from build123d import *

# Parameters (mm, degrees)
SKETCH1_W               = 12.04
SKETCH1_H               = 7.58
SKETCH1_W_2             = 8.04
SKETCH1_H_2             = 3.58
BOSS_EXTRUDE1_DEPTH     = 8
SKETCH1_2_W             = 12.04
SKETCH1_2_H             = 7.58
SKETCH1_2_W_2           = 8.04
SKETCH1_2_H_2           = 3.58
BOSS_EXTRUDE2_DEPTH     = 2
EXTRUDE_THIN1_START     = -12.04
EXTRUDE_THIN1_DEPTH     = 12.04
SKETCH5_W               = 12.04
SKETCH5_H               = 7.58
SKETCH5_W_2             = 8.04
SKETCH5_H_2             = 3.58
BOSS_EXTRUDE4_DEPTH     = 10
SKETCH5_4_W             = 12.04
SKETCH5_4_H             = 7.58
BOSS_EXTRUDE5_DEPTH     = 2
CHAMFER1_SIZE           = 1.5
CUT_EXTRUDE1_DEPTH      = 31.858817668
CUT_EXTRUDE1_DEPTH_BACK = 31.858817668
CUT_EXTRUDE2_DEPTH      = 31.883619629
CUT_EXTRUDE2_DEPTH_BACK = 31.883619629
SKETCH8_W               = 4
SKETCH8_H               = 1.58
CUT_EXTRUDE3_DEPTH      = 7
SKETCH9_W               = 4
SKETCH9_H               = 1.58
CUT_EXTRUDE4_DEPTH      = 7
CHAMFER2_SIZE           = 0.5
BOSS_EXTRUDE6_DEPTH     = 0.3


with BuildPart() as part:
    # Sketch1 → Boss-Extrude1 (new body)
    with BuildSketch(Plane.XY):
        Rectangle(SKETCH1_W, SKETCH1_H)
        Rectangle(SKETCH1_W_2, SKETCH1_H_2, mode=Mode.SUBTRACT)
    extrude(amount=BOSS_EXTRUDE1_DEPTH)

    # Sketch1<2> → Boss-Extrude2 (add)
    # profile 1 of 2: a face of its own
    with BuildSketch(Plane.XY):
        Rectangle(SKETCH1_2_W, SKETCH1_2_H)
        Rectangle(SKETCH1_2_W_2, SKETCH1_2_H_2, mode=Mode.SUBTRACT)
    # profile 2 of 2: a face of its own
    with BuildSketch(Plane.XY):
        Rectangle(SKETCH1_2_W_2, SKETCH1_2_H_2)
    extrude(amount=-BOSS_EXTRUDE2_DEPTH)

    # Sketch3 → Extrude-Thin1 (add)
    with BuildSketch(Plane(origin=(6.02, 9.81, 0), x_dir=(0, -1, 0), z_dir=(1, 0, 0)).offset(EXTRUDE_THIN1_START)):
        with BuildLine():
            Line((13.6, 2), (9.52, 2))
            ThreePointArc((9.52, 2), (9.33452957, 10.5), (8.778471331, 18.983819807))
            Line((8.778471331, 18.983819807), (12.842945699, 19.339415237))
            Line((12.842945699, 19.339415237), (12.668634214, 21.331804633))
            Line((12.668634214, 21.331804633), (6.601440048, 20.800993925))
            ThreePointArc((6.601440048, 20.800993925), (7.336433126, 10.412761225), (7.509629919, 0))
            Line((7.509629919, 0), (13.6, 0))
            Line((13.6, 0), (13.6, 2))
        make_face()
    extrude(amount=EXTRUDE_THIN1_DEPTH)

    # Sketch5 → Boss-Extrude4 (add)
    with BuildSketch(Plane(origin=(0, -2.094837633, -19.257341416), x_dir=(-1, 0, 0), z_dir=(0, 0.08715574274765182, -0.9961946980917462))):
        with Locations((0, 2.848308513)):
            Rectangle(SKETCH5_W, SKETCH5_H)
        with Locations((0, 2.848308513)):
            Rectangle(SKETCH5_W_2, SKETCH5_H_2, mode=Mode.SUBTRACT)
    extrude(amount=BOSS_EXTRUDE4_DEPTH)

    # Sketch5<4> → Boss-Extrude5 (add)
    with BuildSketch(Plane(origin=(0, -2.094837633, -19.257341416), x_dir=(-1, 0, 0), z_dir=(0, 0.08715574274765182, -0.9961946980917462))):
        with Locations((0, 2.848308513)):
            Rectangle(SKETCH5_4_W, SKETCH5_4_H)
    extrude(amount=BOSS_EXTRUDE5_DEPTH)

    # Chamfer1
    chamfer1_edges = [part.edges().sort_by_distance(p)[0] for p in [
        (0, -3.79, -2),
        (0, 3.79, -2),
        (-6.02, -2.597166986, -24.320388728),
        (6.02, -2.597166986, -24.320388728),
        (0, -3.032945699, -19.339415237),
        (6.02, -3.79, 3),
        (-6.02, -3.79, 3),
        (-6.02, 3.79, 3),
        (6.02, 3.79, 3),
        (0, 4.518210112, -18.678774707),
        (6.02, 4.953988826, -23.659748198),
        (-6.02, 4.953988826, -23.659748198),
    ]]
    chamfer(chamfer1_edges, length=CHAMFER1_SIZE - 0.0001)  # a hair under: the kernel refuses the full size

    # Sketch6 → Cut-Extrude1 (cut, two sides: drawn at the far end of the back side and taken through both)
    with BuildSketch(Plane(origin=(0, 3.79, 0), x_dir=(1, 0, 0), z_dir=(0, 1, 0)).offset(-CUT_EXTRUDE1_DEPTH_BACK)):
        with BuildLine():
            Line((1.45, -3.566987298), (-0.35, -2.527756814))
            ThreePointArc((-0.35, -2.527756814), (-0.85, -2.527756814), (-1.1, -2.960769515))
            Line((-1.1, -2.960769515), (-1.1, -5.039230485))
            ThreePointArc((-1.1, -5.039230485), (-0.85, -5.472243186), (-0.35, -5.472243186))
            Line((-0.35, -5.472243186), (1.45, -4.433012702))
            ThreePointArc((1.45, -4.433012702), (1.7, -4), (1.45, -3.566987298))
        make_face()
    extrude(amount=CUT_EXTRUDE1_DEPTH + CUT_EXTRUDE1_DEPTH_BACK, mode=Mode.SUBTRACT)

    # Sketch7 → Cut-Extrude2 (cut, two sides: drawn at the far end of the back side and taken through both)
    with BuildSketch(Plane(origin=(0, 2.862121636, 0.250403197), x_dir=(1, 0, 0), z_dir=(0, 0.9961946980917462, 0.08715574274765181)).offset(-CUT_EXTRUDE2_DEPTH_BACK)):
        with BuildLine():
            Line((1.45, 25.43449699), (-0.35, 26.473727475))
            ThreePointArc((-0.35, 26.473727475), (-0.85, 26.473727475), (-1.1, 26.040714773))
            Line((-1.1, 26.040714773), (-1.1, 23.962253804))
            ThreePointArc((-1.1, 23.962253804), (-0.85, 23.529241102), (-0.35, 23.529241102))
            Line((-0.35, 23.529241102), (1.45, 24.568471587))
            ThreePointArc((1.45, 24.568471587), (1.7, 25.001484288), (1.45, 25.43449699))
        make_face()
    extrude(amount=CUT_EXTRUDE2_DEPTH + CUT_EXTRUDE2_DEPTH_BACK, mode=Mode.SUBTRACT)

    # Sketch8 → Cut-Extrude3 (cut)
    with BuildSketch(Plane(origin=(0, 2.527645904, -28.891124885), x_dir=(-1, 0, 0), z_dir=(0, 0.08715574274765193, -0.9961946980917461))):
        with Locations((-6.02, -0.916945525)):
            Rectangle(SKETCH8_W, SKETCH8_H)
    extrude(amount=-CUT_EXTRUDE3_DEPTH, mode=Mode.SUBTRACT)

    # Sketch9 → Cut-Extrude4 (cut)
    with BuildSketch(Plane.XY.offset(8)):
        with Locations((6.02, 0)):
            Rectangle(SKETCH9_W, SKETCH9_H)
    extrude(amount=-CUT_EXTRUDE4_DEPTH, mode=Mode.SUBTRACT)

    # Chamfer2
    chamfer2_edges = [part.edges().sort_by_distance(p)[0] for p in [
        (4.02, 0.522150723, -25.553213547),
        (4.02, 1.004099435, -21.997679067),
        (4.02, 2.096138346, -25.415507473),
        (4.02, 0.79, 4.5),
        (4.02, 0, 1),
        (4.02, -0.79, 4.5),
    ]]
    chamfer(chamfer2_edges, length=CHAMFER2_SIZE)

    # Sketch10 → Boss-Extrude6 (add)
    with BuildSketch(Plane(origin=(6.02, 0, 0), x_dir=(0, 0, -1), z_dir=(1, 0, 0))):
        with BuildLine():
            Line((21.338592032, 0.15320422), (21.233028007, 1.362426781))
            add(Edge.make_bspline(
                [(21.233028007, 1.362426781), (21.230623172, 1.392016851), (21.22550753, 1.454961769), (21.219940858, 1.554962176), (21.215964545, 1.666017285), (21.21390718, 1.743649504), (21.212829837, 1.784301781)],
                knots=[0, 0, 0, 0, 0.843314449, 1.793924683, 2.844783983, 4, 4, 4, 4], degree=3))
            Line((21.212829837, 1.784301781), (21.202540203, 1.783539585))
            add(Edge.make_bspline(
                [(21.202540203, 1.783539585), (21.200808847, 1.76790896), (21.197498896, 1.738026826), (21.192026096, 1.695375149), (21.187181442, 1.656725646), (21.182258815, 1.622035938), (21.177293915, 1.591439333), (21.172767869, 1.564856175), (21.168316369, 1.542328609), (21.164861999, 1.528700708), (21.163287154, 1.522487756)],
                knots=[0, 0, 0, 0, 1.428769924, 2.731477, 3.906784307, 4.967723303, 5.914548028, 6.722864751, 7.417754754, 8, 8, 8, 8], degree=3))
            Line((21.163287154, 1.522487756), (20.792098129, 0.105567024))
            Line((20.792098129, 0.105567024), (20.453683495, 0.075841415))
            Line((20.453683495, 0.075841415), (19.837067642, 1.393295683))
            add(Edge.make_bspline(
                [(19.837067642, 1.393295683), (19.835006874, 1.398111338), (19.83016149, 1.409434157), (19.822671636, 1.429138703), (19.813894021, 1.454208796), (19.803667873, 1.484424749), (19.792311733, 1.520061222), (19.779237689, 1.560762892), (19.765280196, 1.6069604), (19.755390982, 1.639486413), (19.750177398, 1.656634098)],
                knots=[0, 0, 0, 0, 0.453127431, 1.065416844, 1.823166036, 2.751085321, 3.825012516, 5.058876589, 6.449442438, 8, 8, 8, 8], degree=3))
            Line((19.750177398, 1.656634098), (19.738744471, 1.655490805))
            add(Edge.make_bspline(
                [(19.738744471, 1.655490805), (19.751035456, 1.572245864), (19.77562146, 1.405728657), (19.791432277, 1.238150394), (19.799338983, 1.154347512)],
                knots=[0, 0, 0, 0, 0.999835902, 2, 2, 2, 2], degree=3))
            Line((19.799338983, 1.154347512), (19.898043251, 0.027442024))
            Line((19.898043251, 0.027442024), (19.514659105, -0.006094561))
            Line((19.514659105, -0.006094561), (19.34049752, 1.986283488))
            Line((19.34049752, 1.986283488), (19.957875568, 2.040018244))
            Line((19.957875568, 2.040018244), (20.492555446, 0.873859707))
            add(Edge.make_bspline(
                [(20.492555446, 0.873859707), (20.503235644, 0.85021375), (20.524164125, 0.803878095), (20.550400132, 0.734093054), (20.573588848, 0.666711186), (20.584949885, 0.621787137), (20.59049752, 0.599850561)],
                knots=[0, 0, 0, 0, 1.068017297, 2.092843245, 3.068728431, 4, 4, 4, 4], degree=3))
            Line((20.59049752, 0.599850561), (20.599262764, 0.600612756))
            add(Edge.make_bspline(
                [(20.599262764, 0.600612756), (20.603575304, 0.627567148), (20.611930591, 0.679789657), (20.62621702, 0.755074943), (20.640290752, 0.825113193), (20.651436457, 0.869577883), (20.656808495, 0.891009098)],
                knots=[0, 0, 0, 0, 1.106003676, 2.142815394, 3.104869014, 4, 4, 4, 4], degree=3))
            Line((20.656808495, 0.891009098), (20.983028007, 2.129957268))
            Line((20.983028007, 2.129957268), (21.583637764, 2.182548732))
            Line((21.583637764, 2.182548732), (21.757799349, 0.190170683))
            Line((21.757799349, 0.190170683), (21.338592032, 0.15320422))
        make_face()
    extrude(amount=BOSS_EXTRUDE6_DEPTH)


solid = part.part
Model file for the job. Use its own axes, mm. A direction names the side the tool comes from. Coordinates: 2 decimals unless noted, no trailing zeros. Order: outer loops, then holes, each group sorted by start corner. A loop starts at its lowest first (then second) coordinate and runs counter-clockwise, first axis right, second up. Notation, with made-up numbers: (20.5, 63) -> (65.5, 63) arc R29 cw to (65.5, 95) -> close; hole circle Ø6 at (82, 0.5). An arc over 180 degrees is marked (long way). Return JSON: item names as keys, results as strings. Group by question number.
Item 1: Saw through at B-B on x = 0.5. State how many separate pieces and enclosed holes the cut face has, then the cut area to 3 significant figures.
Item 2: Flat gauge pins, fed straight in: P1, Ø1.9, axis at y = 1, z = -2, coming from the +X side; P2, Ø1.6, axis at x = 5, z = 3.5, coming from the +Y side; P3, Ø1.1, axis at x = -0.5, y = 0.5, coming from the +Z side. Where does each tip first touch, or does it go through?
Item 3: Wall check: line 1 along X through (y, z) = (1, -21.5); line 2 along Z through (x, y) = (1, -2); line 3 along Z through (x, y) = (0.75, 3.5). Give the ranges that are in metal, low to high. Write a range as [from, to].
Item 4: Saw through at C-C on z = -2.5. Write the cut outline in (x, y), then the cut area to 3 significant figures.
Item 5: Pull direction Y, two halves, no side cores. Call faces 4 (the flat face through (1, -3.79, 5)), 5 (the flat face through (1, 1.79, 5)), 6 (the flat face through (-5.26, 4.22, -23.79)): pulls with the +Y half, pulls with the -Y half, needs draft (parallel to the pull), parting line crosses it, or undercut.
Item 6: Tool access for faces 1 (the flat face through (0.95, 2.966, -23.889)), 2 (the flat face through (5, 0.79, 5)), 3 (the cylindrical face through (1.7, -2.8, 4)): list every direction of +Z, -Z, +X, -X, +Y, -Y with a clear straight run to the whole face (end or side of a thin tool).
Values found:
{
 "1": {"separate pieces": "5", "enclosed holes": "0", "area": "108 mm2"},
 "2": {"P1": "stops at x = 6.02", "P2": "stops at y = 3.79", "P3": "stops at z = 0"},
 "3": {"line 1": "x = [-6.02, -4.02], [4.02, 6.32]", "line 2": "z = [-29.29, -25.97], [-24.58, -19.76], [-2, 3.31], [4.69, 8]", "line 3": "z = [-28.81, -25.63], [-23.95, -19.21], [-0.79, 3.16], [4.84, 8]"},
 "4": {"outline": "(-6.02, 0.29) -> (6.02, 0.29) -> (6.02, 2.29) -> (-6.02, 2.29) -> close", "area": "24.1 mm2"},
 "5": {"face 4": "pulls with the -Y half", "face 5": "undercut", "face 6": "pulls with the +Y half"},
 "6": {"face 1": "-Z", "face 2": "+Z, +X", "face 3": "+Y, -Y"}
}
